Geometry: see drawing. Coordinates: mm, zero at the bounding-box minimum. Round coordinates to 2 decimals unless told otherwise and drop trailing zeros. Write each loop counter-clockwise with the first axis right and the second up, starting at its lowest first coordinate (ties: lowest second). Pieces come first, ordered by that corner, then holes. Notation, with made-up numbers: M 39.5,19.25 L 49.5,19.25 A31 ccw 49.5,47.25 Z; hole C 89,1.5 d2. An arc over 180 degrees is marked long. Use a Markdown table: item, result.
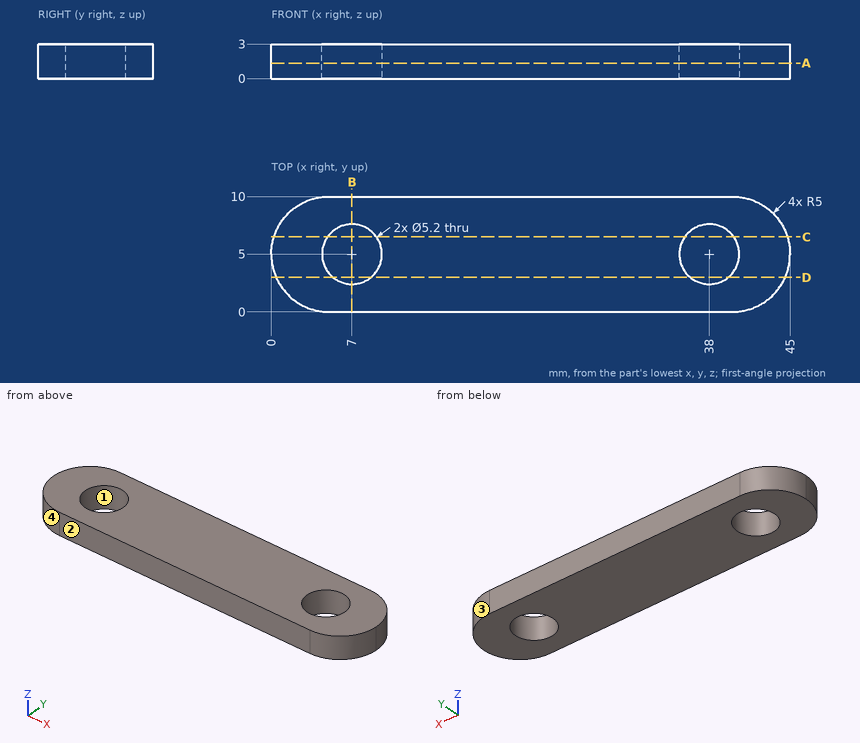
Q1. First-contact query: pin 1 Ø3 at (x, y) = (7, 5) entering from +Z. Flat tip, straight axial feed; report the tip coordinate or a pass-through.
Results are:
| item | result |
|---|---|
| pin 1 | through |
Q2. Section A-A on z = 1.35. Give the number of separate pieces and of enclosed holes in the cut face, plus the area to 3 significant figures.
Results are:
| item | result |
|---|---|
| separate pieces | 1 |
| enclosed holes | 2 |
| area | 386 mm^2 |
Q3. Section B-B on x = 7. Return loops of the section in (y, z).
Results are:
| item | result |
|---|---|
| outline | M 0,0 L 2.4,0 L 2.4,3 L 0,3 Z; M 7.6,0 L 10,0 L 10,3 L 7.6,3 Z |
Q4. Section D-D on y = 3. Return loops of the section in (x, z).
Results are:
| item | result |
|---|---|
| outline | M 0.42,0 L 5.34,0 L 5.34,3 L 0.42,3 Z; M 8.66,0 L 36.34,0 L 36.34,3 L 8.66,3 Z; M 39.66,0 L 44.58,0 L 44.58,3 L 39.66,3 Z |
Q5. Line query: L1, parallel to Y at x = 7, z = 1.6; L2, parallel to X at y = 5.5, z = 0.8 (1 decimal); L3, parallel to X at y = 2.75, z = 1.4 (1 decimal). Output: solid intervals per line, ascending.
Results are:
| item | result |
|---|---|
| L1 | 0 to 2.4, 7.6 to 10 |
| L2 | 0 to 4.4, 9.6 to 35.4, 40.6 to 45 |
| L3 | 0.5 to 5.7, 8.3 to 36.7, 39.3 to 44.5 |
Q6. Mould query, pull axis X, two halves, no side actions, for the marked faces 1, 2, 3 and 4. Classes: +X half, -X half, draft (parallel to the pull), parting line (faces both ways), or undercut.
Results are:
| item | result |
|---|---|
| face 1 | undercut |
| face 2 | draft |
| face 3 | +X half |
| face 4 | -X half |
Q7. Section C-C on y = 6.5. Return loops of the section in (x, z).
Results are:
| item | result |
|---|---|
| outline | M 0.23,0 L 4.88,0 L 4.88,3 L 0.23,3 Z; M 9.12,0 L 35.88,0 L 35.88,3 L 9.12,3 Z; M 40.12,0 L 44.77,0 L 44.77,3 L 40.12,3 Z |
